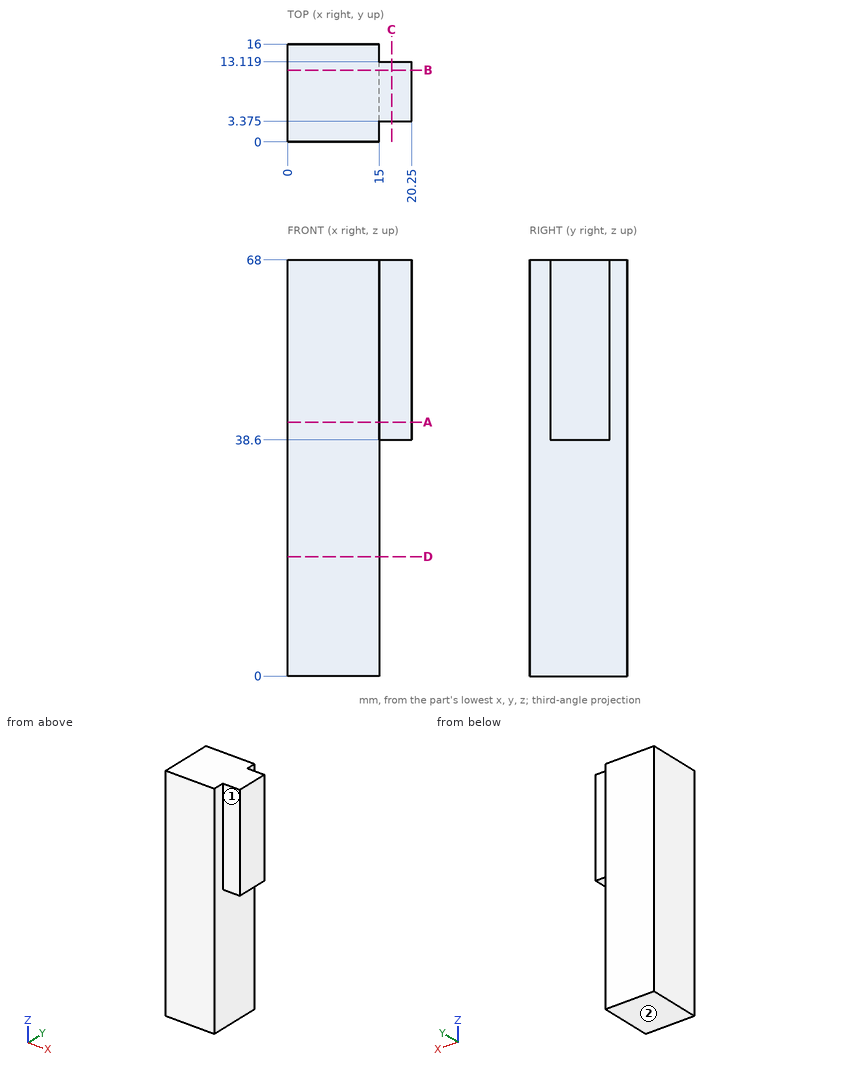
Can you work these out from the drawing? Everything is in mm from the part's minimum corner. A direction names the side the tool comes from. Give positions to 0.01 mm unless a question says otherwise; leave off trailing zeros. Order: outer loops, then holes, each group sorted by start corner. A loop starts at its lowest first (then second) coordinate and runs counter-clockwise, first axis right, second up. Notation, with made-up numbers: M 9.25,58.25 L 55.25,58.25 A18 cw 55.25,79.25 Z; hole C -18,-29.5 d2. An arc over 180 degrees is marked long. Use a Markdown table: item, result. Add a question column.
Item 1: Suppose I cut it at D-D (z = 19.5). List the corners of the cut face in (x, y) for me.
Item 2: If I drill on L1, parallel to X at y = 1.25, z = 9; L2, parallel to Z at x = 16.75, y = 11; L3, parallel to Y at x = 18.5, z = 55.5 (3 decimals), over which ranges is the centre line in solid material (lowest first)? Write a range as [from, to].
Item 3: Will these pins go through, and if not, where does the flat tip stop? pin 1 (5 mm diameter, centred on y = 11.5, z = 35, fed in from +X); pin 2 (2 mm diameter, centred on y = 3, z = 42.5, fed in from +X); pin 3 (4 mm diameter, centred on x = 18, z = 48.5, fed in from -Y) (3 decimals); pin 4 (2.5 mm diameter, centred on x = 17.5, z = 52, fed in from +Y).
Item 4: Suppose I cut it at A-A (z = 41.5). List the corners of the cut face in (x, y) for me (3 decimals), then the cut area to 3 significant figures.
Item 5: For the marked faces 1 and 2, which set-ups out of +Z, -Z, +X, -X, +Y, -Y let a thin tool reach every point of the face, with its end or its side?
Item 6: Suppose I cut it at B-B (y = 11.75). List the corners of the cut face in (x, z) for me, then the cut area to 3 significant figures.
Item 7: Suppose I cut it at C-C (x = 17). List the corners of the cut face in (y, z) for me (3 decimals), then the cut area to 3 significant figures.
Answer sheet:
| question | item | result |
|---|---|---|
| 1 | outline | M 0,0 L 15,0 L 15,16 L 0,16 Z |
| 2 | L1 | x = [0, 15] |
| 2 | L2 | z = [38.6, 68] |
| 2 | L3 | y = [3.375, 13.119] |
| 3 | pin 1 | stops at x = 15 |
| 3 | pin 2 | stops at x = 20.25 |
| 3 | pin 3 | stops at y = 3.375 |
| 3 | pin 4 | stops at y = 13.12 |
| 4 | outline | M 0,0 L 15,0 L 15,3.375 L 20.25,3.375 L 20.25,13.119 L 15,13.119 L 15,16 L 0,16 Z |
| 4 | area | 291 mm² |
| 5 | face 1 | +Z, -Z, +X, -Y |
| 5 | face 2 | -Z, +X, -X, +Y, -Y |
| 6 | outline | M 0,0 L 15,0 L 15,38.6 L 20.25,38.6 L 20.25,68 L 0,68 Z |
| 6 | area | 1,170 mm² |
| 7 | outline | M 3.375,38.6 L 13.119,38.6 L 13.119,68 L 3.375,68 Z |
| 7 | area | 286 mm² |
